```python
from build123d import *

# Parameters (mm, degrees)
SKETCH1_W           = 30
SKETCH1_H           = 40
BOSS_EXTRUDE1_DEPTH = 2
FILLET1_R           = 2
SKETCH2_R           = 1.25
BOSS_EXTRUDE2_DEPTH = 4
BOSS_EXTRUDE3_START = 2
BOSS_EXTRUDE3_DEPTH = 2


with BuildPart() as part:
    # Sketch1 → Boss-Extrude1 (new body)
    with BuildSketch(Plane.XY):
        with Locations((-68.585871194, -180)):
            Rectangle(SKETCH1_W, SKETCH1_H)
    extrude(amount=BOSS_EXTRUDE1_DEPTH)

    # Fillet1
    fillet1_edges = [part.edges().sort_by_distance(p)[0] for p in [
        (-83.585871194, -160, 1),
        (-53.585871194, -160, 1),
        (-53.585871194, -200, 1),
        (-83.585871194, -200, 1),
    ]]
    fillet(fillet1_edges, radius=FILLET1_R)

    # Sketch2 → Boss-Extrude2 (add)
    with BuildSketch(Plane.XY.offset(2)):
        with Locations((-81.085871194, -197.5)):
            Circle(SKETCH2_R)
        with Locations(Location((-56.085871194, -197.5, 0), (0, 0, 180))):
            Circle(SKETCH2_R)
        with Locations((-56.085871194, -162.5)):
            Circle(SKETCH2_R)
        with Locations(Location((-81.085871194, -162.5, 0), (0, 0, 180))):
            Circle(SKETCH2_R)
    extrude(amount=BOSS_EXTRUDE2_DEPTH)

    # Sketch3 → Boss-Extrude3 (add)
    with BuildSketch(Plane.XY.offset(6).offset(BOSS_EXTRUDE3_START)):
        with BuildLine():
            Line((-53.585871194, -198), (-53.585871194, -162))
            ThreePointArc((-53.585871194, -162), (-54.171657631, -160.585786438), (-55.585871194, -160))
            Line((-55.585871194, -160), (-81.585871194, -160))
            ThreePointArc((-81.585871194, -160), (-83.000084756, -160.585786438), (-83.585871194, -162))
            Line((-83.585871194, -162), (-83.585871194, -198))
            ThreePointArc((-83.585871194, -198), (-83.000084756, -199.414213562), (-81.585871194, -200))
            Line((-81.585871194, -200), (-55.585871194, -200))
            ThreePointArc((-55.585871194, -200), (-54.171657631, -199.414213562), (-53.585871194, -198))
        make_face()
    extrude(amount=-BOSS_EXTRUDE3_DEPTH)


solid = part.part
```
The model under review builds one solid part; all positions refer to its coordinate system, in mm. A direction names the side the tool comes from. Round coordinates to 2 decimals unless told otherwise and drop trailing zeros. Order: outer loops, then holes, each group sorted by start corner. A loop starts at its lowest first (then second) coordinate and runs counter-clockwise, first axis right, second up. Notation, with made-up numbers: (-1.75, 29.5) - (46.25, 29.5) arc R18 ccw to (46.25, 38.5) - close; hole circle Ø11 at (61, -29). An arc over 180 degrees is marked (long way). Answer in a Markdown table with one row per item.
(1) Machinability: for faces 1 (the face through (-81.36, -198.72, 3.97)), 2 (the face through (-83.016, -160.601, 1.014)), which of the approach directions +Z, -Z, +X, -X, +Y, -Y give a long, thin tool a straight path to every point of the face, cutting with its end or side? Answer none if there is none.
Result set:
| item | result |
|---|---|
| face 1 | none |
| face 2 | +Z, -Z, -X, +Y |
(2) For line 1 (Z direction, x = -58, y = -185.5); line 2 (Y direction, x = -80, z = 5); line 3 (Y direction, x = -82, z = 6.75), list the stretches that pass through material, from the lowest coordinate up. Write a range as from..to.
Result set:
| item | result |
|---|---|
| line 1 | z = 0..2, 6..8 |
| line 2 | y = -198.12..-196.88, -163.12..-161.88 |
| line 3 | y = -199.96..-160.04 |
(3) Take a section at D-D on x = -81. Write out the cut boundary in (y, z).
Result set:
| item | result |
|---|---|
| outline | (-200, 0) - (-160, 0) - (-160, 2) - (-161.25, 2) - (-161.25, 6) - (-160, 6) - (-160, 8) - (-200, 8) - (-200, 6) - (-198.75, 6) - (-198.75, 2) - (-200, 2) - close; hole (-196.25, 2) - (-163.75, 2) - (-163.75, 6) - (-196.25, 6) - close |
(4) Take a section at A-A on y = -184. Write out the cut boundary in (x, z).
Result set:
| item | result |
|---|---|
| outline | (-83.59, 0) - (-53.59, 0) - (-53.59, 2) - (-83.59, 2) - close; (-83.59, 6) - (-53.59, 6) - (-53.59, 8) - (-83.59, 8) - close |
(5) Clearance check with flat-ended pins moving along their axes: P1, Ø2, axis at x = -62.5, y = -173, coming from the -Z side; P2, Ø1.5, axis at x = -79, z = 5, coming from the +Y side. State where each tip first meets the part, or that it passes through.
Result set:
| item | result |
|---|---|
| P1 | stops at z = 0 |
| P2 | passes through |
(6) Take a section at B-B on x = -59. Write out the cut boundary in (y, z).
Result set:
| item | result |
|---|---|
| outline | (-200, 0) - (-160, 0) - (-160, 2) - (-200, 2) - close; (-200, 6) - (-160, 6) - (-160, 8) - (-200, 8) - close |
(7) Mouldability with a two-part tool opening along Y and no side actions: class faces 3 (the face through (-69, -200, 1)), 4 (the face through (-69, -180, 6)), 5 (the face through (-53.586, -180, 7)) as released by +Y, released by -Y, zero draft, split by the parting line, or undercut.
Result set:
| item | result |
|---|---|
| face 3 | released by -Y |
| face 4 | undercut |
| face 5 | zero draft |
(8) Take a section at C-C on y = -162.5. Write out the cut boundary in (x, z), plus the area to 3 significant figures.
Result set:
| item | result |
|---|---|
| outline | (-83.59, 0) - (-53.59, 0) - (-53.59, 2) - (-54.84, 2) - (-54.84, 6) - (-53.59, 6) - (-53.59, 8) - (-83.59, 8) - (-83.59, 6) - (-82.34, 6) - (-82.34, 2) - (-83.59, 2) - close; hole (-79.84, 2) - (-57.34, 2) - (-57.34, 6) - (-79.84, 6) - close |
| area | 140 mm2 |
